Job drawing, mm, ordinate dimensions from the low corner. One solid piece. Round coordinates to 2 decimals unless told otherwise and drop trailing zeros. Write each loop counter-clockwise with the first axis right and the second up, starting at its lowest first coordinate (ties: lowest second). Pieces come first, ordered by that corner, then holes.
1) Saw through at B-B (z = 25.5). Write the cut outline in (x, y).
2) Wall check: probe 1 along Z at (x, y) = (2.5, 3.4); probe 2 along X at (y, z) = (3.3, 25.5); probe 3 along X at (y, z) = (0.4, 11.5). Give the ranges that are in metal, low to high.
3) Pull direction Z, two halves, no side cores. Call the marked faces 1, 2 and 3: +Z half, -Z half, draft (parallel to the pull), parting line (faces both ways), or undercut.
4) Flat gauge pins, fed straight in: pin 1 (1.4 mm diameter, centred on x = 37.5, z = 25.5, fed in from +Y); pin 2 (3 mm diameter, centred on x = 2.5, z = 10.5, fed in from -Y); pin 3 (4 mm diameter, centred on x = 2.5, z = 25.5, fed in from -Y); pin 4 (4.5 mm diameter, centred on x = 27.5, z = 18, fed in from +Y). Where does each tip first touch, or does it go through?
5) Saw through at D-D (y = 2.15). Write the cut outline in (x, z).
6) Saw through at A-A (x = 37.5). Write the cut outline in (y, z).
7) Saw through at C-C (x = 12.5). Write the cut outline in (y, z), plus the area to 3 significant figures.
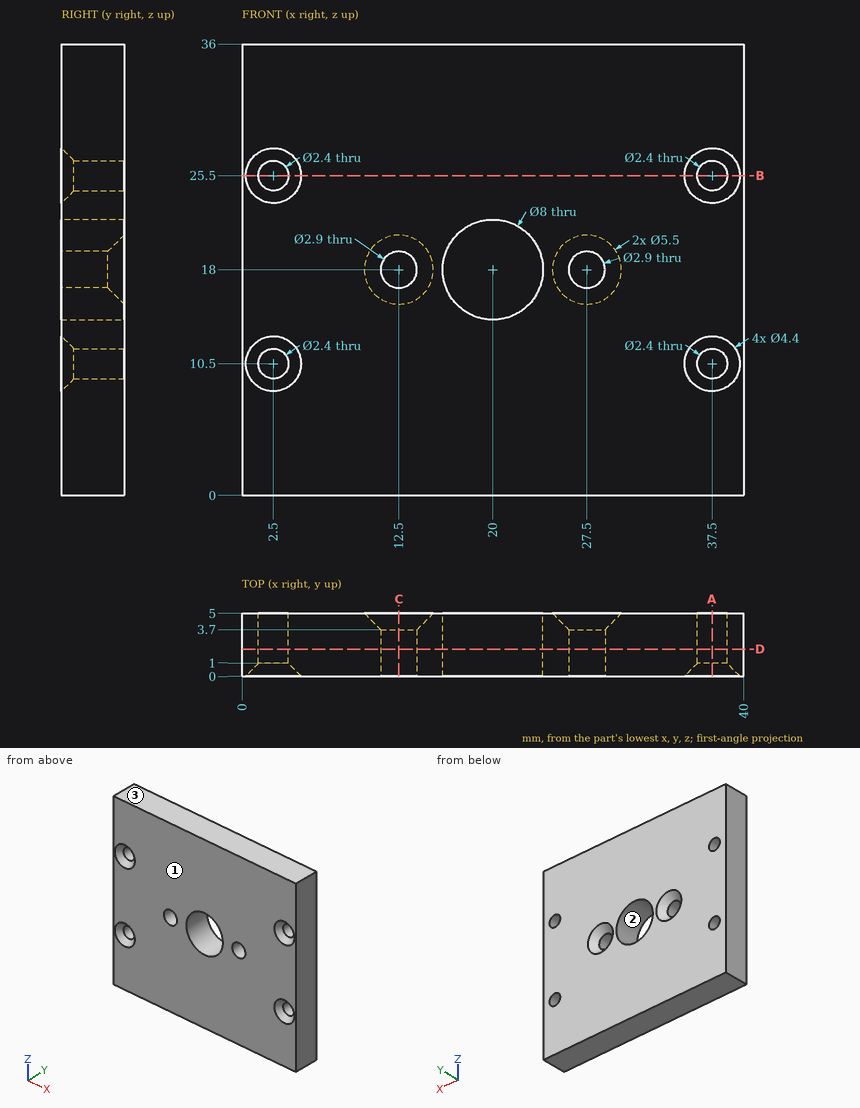
Evaluation:
1. outline: (0, 0) - (0.3, 0) - (1.3, 1) - (1.3, 5) - (0, 5) - close; (3.7, 1) - (4.7, 0) - (35.3, 0) - (36.3, 1) - (36.3, 5) - (3.7, 5) - close; (38.7, 1) - (39.7, 0) - (40, 0) - (40, 5) - (38.7, 5) - close
2. probe 1: z = 0 to 9.3, 11.7 to 24.3, 26.7 to 36
2. probe 2: x = 0 to 1.3, 3.7 to 36.3, 38.7 to 40
2. probe 3: x = 0 to 1, 4 to 36, 39 to 40
3. face 1: draft
3. face 2: undercut
3. face 3: +Z half
4. pin 1: passes through
4. pin 2: stops at y = 0.7
4. pin 3: stops at y = 0.2
4. pin 4: stops at y = 4.5
5. outline: (0, 0) - (40, 0) - (40, 36) - (0, 36) - close; hole circle Ø2.4 at (2.5, 10.5); hole circle Ø2.4 at (2.5, 25.5); hole circle Ø2.9 at (12.5, 18); hole circle Ø8 at (20, 18); hole circle Ø2.9 at (27.5, 18); hole circle Ø2.4 at (37.5, 10.5); hole circle Ø2.4 at (37.5, 25.5)
6. outline: (0, 0) - (5, 0) - (5, 9.3) - (1, 9.3) - (0, 8.3) - close; (0, 12.7) - (1, 11.7) - (5, 11.7) - (5, 24.3) - (1, 24.3) - (0, 23.3) - close; (0, 27.7) - (1, 26.7) - (5, 26.7) - (5, 36) - (0, 36) - close
7. outline: (0, 0) - (5, 0) - (5, 15.25) - (3.7, 16.55) - (0, 16.55) - close; (0, 19.45) - (3.7, 19.45) - (5, 20.75) - (5, 36) - (0, 36) - close
7. area: 164 mm2
